Build history of the part. All positions in model axes, mm. Face numbers are marked on the shaded views. A direction names the side the tool comes from. Give positions to 0.01 mm unless a question says otherwise; leave off trailing zeros. Order: outer loops, then holes, each group sorted by start corner. A loop starts at its lowest first (then second) coordinate and runs counter-clockwise, first axis right, second up. Notation, with made-up numbers: (-18, 83.5) -> (5, 83.5) arc R16 ccw to (5, 109.5) -> close; hole circle Ø5 at (80.5, 16.25). An arc over 180 degrees is marked (long way). One line per question, with ' | ' between items. Start each with the question number.
(1) Which spindle directions (+Z, -Z, +X, -X, +Y, -Y) get a long thin tool onto all of the face, cutting with end or side? Do the marked faces 3 and 4. Say none if no direction does.
(2) Cut at B-B (z = -6). Give the cut face in (x, y).
(3) Cut at A-A (z = -3.25). Give the cut face in (x, y), then the cut area to 3 significant figures.
(4) Pin check, flat tips, straight feed: pin 1 Ø3 at (y, z) = (5, 6.5) entering from +X; pin 2 Ø1 at (y, z) = (10, 0) entering from -X; pin 3 Ø8 at (x, z) = (0, 0) entering from -Y; pin 4 Ø1.5 at (y, z) = (4, -1.5) entering from +X. Stop position of each tip, or through.
(5) Drill centre lines: L1, parallel to Y at x = 5.5, z = 0; L2, parallel to Z at x = 5.5, y = 1 (3 decimals); L3, parallel to X at y = 1.75, z = 5.75. Where is each one in solid material? Low to high. Write a range as from..to.
(6) Pull direction Z, two halves, no side cores. Call the marked faces 1 and 2: +Z half, -Z half, draft (parallel to the pull), parting line (faces both ways), or undercut.
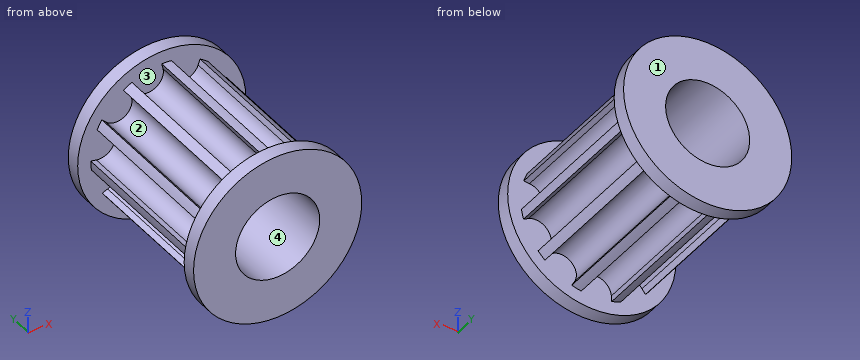
Autodesk Inventor part; units mm, degrees
ref_plane "YZ Plane" through (0, 0, 0) normal (1, 0, 0) x (0, 1, 0)
ref_plane "XZ Plane" through (0, 0, 0) normal (0, 1, 0) x (-1, 0, 0)
ref_plane "XY Plane" through (0, 0, 0) normal (0, 0, 1) x (1, 0, 0)
sketch "Esquisse2" plane through (0, 0, 0) normal (0, 1, 0) x (-1, 0, 0)
  circle A0 centre (0, 0) radius 7.6
  dimension "d0" = 15.2
extrude "Extrusion1" add sketch "Esquisse2" along normal blind 17
sketch "Esquisse4" plane through (0, 17, 0) normal (0, 1, 0) x (1, 0, 0)
  circle A0 centre (0, 0) radius 7.6
  circle A1 centre (0, 0) radius 7.6
  arc A2 (-3.2, -6.8935) -> (0, -7.6) centre (0, 0) ccw
  line L0 (-0.0062, -0.0113) -> (-4.6214, -8.4012)
  line L1 (0, -6.3735) -> (0, 5.2233) construction
  line L2 (-3.2, -6.8935) -> (0, -7.6) construction
  line L3 (-3.2, -6.8935) -> (-3.0675, -6.2935)
  line L4 (0, -7.6) -> (0.1325, -7)
  arc A3 (0.1325, -7) -> (-3.0675, -6.2935) centre (-1.4675, -6.6467) ccw
  line L5 (-3.0675, -6.2935) -> (0.1325, -7) construction
  arc A4 (-6.419, -4.069) -> (-4.109, -6.3935) centre (0, 0) ccw
  line L6 (-4.109, -6.3935) -> (-6.419, -4.069) construction
  line L7 (-4.109, -6.3935) -> (-3.6731, -5.9603)
  line L8 (-6.419, -4.069) -> (-5.9831, -3.6359)
  arc A5 (-3.6731, -5.9603) -> (-5.9831, -3.6359) centre (-4.8281, -4.7981) ccw
  line L9 (-3.6731, -5.9603) -> (-5.9831, -3.6359) construction
  line L10 (-4.109, -6.3935) -> (-3.2, -6.8935) construction
  line L11 (0, 0) -> (-8.9658, -4.8594)
  arc A6 (-6.3677, 4.1487) -> (-7.5226, 1.0819) centre (0, 0) ccw
  line L12 (-7.5226, 1.0819) -> (-6.3677, 4.1487) construction
  line L13 (-7.5226, 1.0819) -> (-6.9476, 0.8653)
  line L14 (-6.3677, 4.1487) -> (-5.7927, 3.9322)
  arc A7 (-6.9476, 0.8653) -> (-5.7927, 3.9322) centre (-6.3701, 2.3988) ccw
  line L15 (-6.9476, 0.8653) -> (-5.7927, 3.9322) construction
  arc A8 (-7.5999, 0.0474) -> (-6.9133, -3.157) centre (0, 0) ccw
  line L16 (-7.5999, 0.0474) -> (-6.9133, -3.157) construction
  line L17 (-7.5999, 0.0474) -> (-6.999, 0.1761)
  line L18 (-6.9133, -3.157) -> (-6.3125, -3.0282)
  arc A9 (-6.3125, -3.0282) -> (-6.999, 0.1761) centre (-6.6558, -1.4261) ccw
  line L19 (-6.999, 0.1761) -> (-6.3125, -3.0282) construction
  line L20 (-7.5999, 0.0474) -> (-7.5226, 1.0819) construction
  line L21 (-6.9133, -3.157) -> (-6.419, -4.069) construction
  line L22 (0, 0) -> (-6.7758, 5.1057)
  arc A10 (7.3055, 2.0952) -> (5.7441, 4.9764) centre (0, 0) ccw
  line L23 (5.7441, 4.9764) -> (7.3055, 2.0952) construction
  line L24 (5.7441, 4.9764) -> (5.2039, 4.6837)
  line L25 (7.3055, 2.0952) -> (6.7653, 1.8025)
  arc A11 (5.2039, 4.6837) -> (6.7653, 1.8025) centre (5.9846, 3.2431) ccw
  line L26 (5.2039, 4.6837) -> (6.7653, 1.8025) construction
  arc A12 (5.0129, 5.7123) -> (2.1417, 7.292) centre (0, 0) ccw
  line L27 (5.0129, 5.7123) -> (2.1417, 7.292) construction
  line L28 (5.0129, 5.7123) -> (4.7167, 5.174)
  line L29 (2.1417, 7.292) -> (1.8455, 6.7536)
  arc A13 (1.8455, 6.7536) -> (4.7167, 5.174) centre (3.2811, 5.9638) ccw
  line L30 (4.7167, 5.174) -> (1.8455, 6.7536) construction
  line L31 (5.0129, 5.7123) -> (5.7441, 4.9764) construction
  line L32 (-3.1138, 6.9328) -> (-2.7472, 6.4398)
  arc A14 (-5.3768, 4.4842) -> (-2.7472, 6.4398) centre (-4.062, 5.462) ccw
  line L33 (-2.7472, 6.4398) -> (-5.3768, 4.4842) construction
  line L34 (-3.1138, 6.9328) -> (-5.7434, 4.9772) construction
  arc A15 (-3.1138, 6.9328) -> (-5.7434, 4.9772) centre (0, 0) ccw
  line L35 (-5.7434, 4.9772) -> (-5.3768, 4.4842)
  line L36 (-2.1407, 7.2923) -> (-3.1138, 6.9328) construction
  line L37 (-2.1407, 7.2923) -> (-2.0988, 6.6793)
  line L38 (-2.0988, 6.6793) -> (1.1706, 6.9027) construction
  line L39 (-2.1407, 7.2923) -> (1.1287, 7.5157) construction
  arc A16 (1.1287, 7.5157) -> (-2.1407, 7.2923) centre (0, 0) ccw
  arc A17 (-2.0988, 6.6793) -> (1.1706, 6.9027) centre (-0.4641, 6.791) ccw
  line L40 (1.1287, 7.5157) -> (1.1706, 6.9027)
  line L41 (1.1287, 7.5157) -> (2.1417, 7.292) construction
  line L42 (-6.3677, 4.1487) -> (-5.7434, 4.9772) construction
  line L43 (0, 0) -> (10.678, -14.3583) construction
  arc A18 (7.2785, -2.1871) -> (7.5228, 1.0808) centre (0, 0) ccw
  line L44 (7.5228, 1.0808) -> (7.2785, -2.1871) construction
  line L45 (7.5228, 1.0808) -> (6.91, 1.1266)
  line L46 (7.2785, -2.1871) -> (6.6658, -2.1413)
  arc A19 (6.91, 1.1266) -> (6.6658, -2.1413) centre (6.7879, -0.5073) ccw
  line L47 (6.91, 1.1266) -> (6.6658, -2.1413) construction
  line L48 (7.3055, 2.0952) -> (7.5228, 1.0808) construction
  line L49 (7.2785, -2.1871) -> (0, -7.6) construction
  line L50 (0, 0) -> (10.2791, -3.8716)
  line L51 (1.0339, -7.5293) -> (0.8211, -6.9529)
  arc A20 (3.8952, -5.8176) -> (0.8211, -6.9529) centre (2.3581, -6.3853) ccw
  arc A21 (1.0339, -7.5293) -> (4.1081, -6.394) centre (0, 0) ccw
  line L52 (4.1081, -6.394) -> (3.8952, -5.8176)
  line L53 (0.8211, -6.9529) -> (3.8952, -5.8176) construction
  line L54 (4.9405, -5.775) -> (4.4498, -5.4052)
  arc A22 (6.4221, -2.7881) -> (4.4498, -5.4052) centre (5.436, -4.0967) ccw
  line L55 (4.4498, -5.4052) -> (6.4221, -2.7881) construction
  line L56 (4.9405, -5.775) -> (6.9128, -3.1579) construction
  arc A23 (4.9405, -5.775) -> (6.9128, -3.1579) centre (0, 0) ccw
  line L57 (6.9128, -3.1579) -> (6.4221, -2.7881)
  line L58 (7.2785, -2.1871) -> (6.9128, -3.1579) construction
  point P0 (-7.5999, 0.0474)
  point P1 (-6.9133, -3.157)
  point P2 (-6.3677, 4.1487)
  point P3 (-7.5226, 1.0819)
  point P4 (-3.1138, 6.9328)
  point P5 (-5.7434, 4.9772)
  point P6 (1.1287, 7.5157)
  point P7 (-2.1407, 7.2923)
  point P8 (5.0129, 5.7123)
  point P9 (2.1417, 7.292)
  point P10 (7.3055, 2.0952)
  point P11 (5.7441, 4.9764)
  point P12 (-3.2, -6.8935)
  point P13 (0, -7.6)
  point P14 (-6.419, -4.069)
  point P15 (-4.109, -6.3935)
  point P16 (7.2785, -2.1871)
  point P17 (7.5228, 1.0808)
  point P18 (4.9405, -5.775)
  point P19 (4.9405, -5.775)
  point P20 (6.9128, -3.1579)
  point P21 (1.0339, -7.5293)
  point P22 (4.1081, -6.394)
  dimension "d14" = 3.2
  dimension "d28" = 0.6
  dimension "d30" = 0.5
extrude "Extrusion6" cut sketch "Esquisse4" against normal through all contours A0 L46 A19 L45 | L25 A11 L24 A0 | A0 L54 A22 L57 | L28 A13 L29 A0 | A0 L51 A20 L52 | A0 L17 A9 L18 | L8 A5 L7 A0 | A0 L32 A14 L35 | L14 A7 L13 A0 | L40 A17 L37 A0 | A0 L3 A3 L4
sketch "Esquisse6" plane through (0, 17, 0) normal (0, 1, 0) x (1, 0, 0)
  circle A0 centre (0, 0) radius 9
  dimension "d19" = 18
extrude "Extrusion3" add sketch "Esquisse6" along normal blind 1.5
sketch "Esquisse7" plane through (0, 0, 0) normal (0, -1, 0) x (1, 0, 0)
  circle A0 centre (0, 0) radius 9
  dimension "d34" = 18
extrude "Extrusion4" add sketch "Esquisse7" along normal blind 1.5
sketch "Esquisse8" plane through (0, 18.5, 0) normal (0, 1, 0) x (1, 0, 0)
  circle A0 centre (0, 0) radius 4.5
  dimension "d24" = 9
extrude "Extrusion5" cut sketch "Esquisse8" against normal through all
properties part number "Pièce_moteur_courroie_test_6"
Result set:
1) face 3: none | face 4: +Y, -Y
2) outline: (-6.71, -1.5) -> (6.71, -1.5) -> (6.71, 0) -> (1.64, 0) -> (1.64, 17) -> (6.71, 17) -> (6.71, 18.5) -> (-6.71, 18.5) -> (-6.71, 17) -> (-2.51, 17) -> (-2.51, 0) -> (-6.71, 0) -> close; hole (-1.9, 0) -> (0.97, 0) -> (0.97, 17) -> (-1.9, 17) -> close
3) outline: (-8.39, -1.5) -> (-3.11, -1.5) -> (-3.11, 18.5) -> (-8.39, 18.5) -> (-8.39, 17) -> (-4.97, 17) -> (-4.97, 0) -> (-8.39, 0) -> close; (3.11, -1.5) -> (8.39, -1.5) -> (8.39, 0) -> (4.35, 0) -> (4.35, 17) -> (8.39, 17) -> (8.39, 18.5) -> (3.11, 18.5) -> close | area: 84.2 mm2
4) pin 1: stops at x = 4.94 | pin 2: stops at x = -7.6 | pin 3: passes through | pin 4: stops at x = 7.52
5) L1: y = -1.5..0, 17..18.5 | L2: z = -5.245..-4.844, -1.678..-0.506, 1.52..2.459 | L3: x = -3.49..-2.84, -0.1..0.85, 3.87..4.91
6) face 1: draft | face 2: undercut
